from build123d import *

# Parameters (mm, degrees)
RESSALTO_EXTRUS_O2_DEPTH = 20
ESBO_O3_R                = 13.75
BOSS_EXTRUDE1_DEPTH      = 10
SKETCH2_R                = 2.5
BOSS_EXTRUDE2_DEPTH      = 5
CUT_EXTRUDE2_DEPTH       = 20


with BuildPart() as part:
    # Esboço1 → Ressalto-extrusão2 (new body)
    with BuildSketch(Plane(origin=(0, 0, 0), x_dir=(1, 0, 0), z_dir=(0, 1, 0))):
        with BuildLine():
            ThreePointArc((-12.375, -21.434128744), (0, -24.75), (12.375, -21.434128744))
            ThreePointArc((12.375, -21.434128744), (21.434128744, -12.375), (24.75, 0))
            ThreePointArc((24.75, 0), (-12.375, 21.434128744), (-12.375, -21.434128744))
        make_face()
    extrude(amount=RESSALTO_EXTRUS_O2_DEPTH)

    # Esboço3 → Boss-Extrude1 (add)
    with BuildSketch(Plane(origin=(0, 20, 0), x_dir=(1, 0, 0), z_dir=(0, 1, 0))):
        Circle(ESBO_O3_R)
    extrude(amount=BOSS_EXTRUDE1_DEPTH)

    # Sketch2 → Boss-Extrude2 (add)
    with BuildSketch(Plane(origin=(0, 30, 0), x_dir=(1, 0, 0), z_dir=(0, 1, 0))):
        Circle(SKETCH2_R)
        with Locations((9, 0)):
            Circle(SKETCH2_R)
    extrude(amount=BOSS_EXTRUDE2_DEPTH)

    # Sketch3 → Cut-Extrude2 (cut)
    with BuildSketch(Plane(origin=(0, 20, 0), x_dir=(1, 0, 0), z_dir=(0, 1, 0))):
        with BuildLine():
            Line((8.185723081, -18.248121483), (6.13929231, -13.686091112))
            ThreePointArc((6.13929231, -13.686091112), (15, 0), (6.13929231, 13.686091112))
            Line((6.13929231, 13.686091112), (8.185723081, 18.248121483))
            ThreePointArc((8.185723081, 18.248121483), (20, 0), (8.185723081, -18.248121483))
        make_face()
    extrude(amount=-CUT_EXTRUDE2_DEPTH, mode=Mode.SUBTRACT)


solid = part.part
For this review, take the finished solid that the model builds, in its own axes (mm). A direction names the side the tool comes from. Give positions to 0.01 mm unless a question says otherwise; leave off trailing zeros. Order: outer loops, then holes, each group sorted by start corner. A loop starts at its lowest first (then second) coordinate and runs counter-clockwise, first axis right, second up. Notation, with made-up numbers: (-27.5, -32) - (-17.5, -32) arc R29 ccw to (-17.5, 6) - close; hole circle Ø11 at (89, 30). An arc over 180 degrees is marked (long way). Answer as a JSON object with one key per item and string values. Group by question number.
Item 1: Clearance check with flat-ended pins moving along their axes: pin 1 Ø4 at (x, y) = (-9, 11) entering from +Z; pin 2 Ø3 at (x, z) = (13, 4) entering from +Y; pin 3 Ø10 at (x, z) = (-0.5, -12.5) entering from -Y; pin 4 Ø6 at (x, z) = (-9, 18) entering from +Y. State where each tip first meets the part, or that it passes through.
Item 2: Draft analysis for pull direction X (two halves, no side actions). For faces 1 (the cylindrical face through (-2.981, 24.93, 13.423)), 2 (the cylindrical face through (20, 10, 0)), 3 (the flat face through (9, 35, 0)), 4 (the flat face through (7.15, 10.14, -15.94)), state which applies: pulls with the +X half, pulls with the -X half, needs draft (parallel to the pull), parting line crosses it, or undercut.
Item 3: Take a section at A-A on y = 4. Give the boundary of the cut face in (x, z) (3 decimals).
Item 4: Machinability: for faces 5 (the cylindrical face through (6.5, 32.5, -0.1)), 6 (the flat face through (0, 0, 0)), 7 (the cylindrical face through (15, 10, 0)), which of the approach directions +Z, -Z, +X, -X, +Y, -Y give a long, thin tool a straight path to every point of the face, cutting with its end or side? Answer none if there is none.
Item 5: Take a section at D-D on x = 16.5. Give the boundary of the cut face in (y, z), and give its area (3 significant figures).
Item 6: Take a section at C-C on z = 13. Give the boundary of the cut face in (x, y).
Item 7: Wall thickness on line 1 along Y through (x, z) = (-3, 4); line 2 along Y through (x, z) = (-8, -15); line 3 along X through (y, z) = (8, 2): over which ranges is each line inside the solid? List them lowest first.
Item 8: Take a section at B-B on x = 0. Give the boundary of the cut face in (y, z), and give its area (3 significant figures).
Reported:
{
 "1": {"pin 1": "z = 23.74", "pin 2": "y = 30", "pin 3": "y = 0", "pin 4": "y = 20"},
 "2": {"face 1": "parting line crosses it", "face 2": "undercut", "face 3": "needs draft", "face 4": "undercut"},
 "3": {"outline": "circle Ø49.5 at (0, 0); hole (6.139, -13.686) - (8.186, -18.248) arc R20 ccw to (8.186, 18.248) - (6.139, 13.686) arc R15 cw to start"},
 "4": {"face 5": "+Y", "face 6": "+Z, -Z, +X, -X, -Y", "face 7": "+Y, -Y"},
 "5": {"outline": "(0, -18.45) - (20, -18.45) - (20, -11.3) - (0, -11.3) - close; (0, 11.3) - (20, 11.3) - (20, 18.45) - (0, 18.45) - close", "area": "286 mm^2"},
 "6": {"outline": "(-21.06, 0) - (7.48, 0) - (7.48, 20) - (4.48, 20) - (4.48, 30) - (-4.48, 30) - (-4.48, 20) - (-21.06, 20) - close; (15.2, 0) - (21.06, 0) - (21.06, 20) - (15.2, 20) - close"},
 "7": {"line 1": "0 to 30", "line 2": "0 to 20", "line 3": "-24.67 to 14.87, 19.9 to 24.67"},
 "8": {"outline": "(0, -24.75) - (20, -24.75) - (20, -13.75) - (30, -13.75) - (30, -2.5) - (35, -2.5) - (35, 2.5) - (30, 2.5) - (30, 13.75) - (20, 13.75) - (20, 24.75) - (0, 24.75) - close", "area": "1,290 mm^2"}
}
